Source: CAD feature listing. Evaluate the final solid. Frame: model axes, mm. Face numbers are marked on the shaded views. A direction names the side the tool comes from. Coordinates: 2 decimals unless noted, no trailing zeros. Write each loop counter-clockwise with the first axis right and the second up, starting at its lowest first coordinate (ties: lowest second). Pieces come first, ordered by that corner, then holes. Notation, with made-up numbers: M -36.75,11 L 0.25,11 A20 ccw 0.25,50 Z; hole C -36,50.5 d10. An arc over 180 degrees is marked long. Write item = value, one per line. Start each with the question number.
1. Pull-direction query (Y, two-part tool) for the marked faces 4, 5 and 6; classes: pulls with the +Y half, pulls with the -Y half, needs draft (parallel to the pull), parting line crosses it, or undercut.
2. Section query C-C (x = -10.5). Output: boundary loops of the cut face in (y, z), then the cut area to 3 significant figures.
3. Pin query (flat end, axial travel): pin 1 Ø5 at (x, z) = (-30, -24) entering from -Y; pin 2 Ø8 at (y, z) = (23.5, 6) entering from -X; pin 3 Ø3 at (x, z) = (-31, 23.5) entering from +Y; pin 4 Ø7 at (x, z) = (-9, -25.5) entering from +Y. Return the tip coordinate at first contact, or that it passes through.
4. Line query: line 1 along Z through (x, y) = (-10, -1); line 2 along Z through (x, y) = (5, 9.05); line 3 along Z through (x, y) = (-10, -5). Output: solid intervals per line, ascending.
5. Section query D-D (x = -5). Output: boundary loops of the cut face in (y, z), then the cut area to 3 significant figures.
6. Access query for the marked faces 1, 2 and 3. Directions: +Z, -Z, +X, -X, +Y, -Y. A direction counts if a zero-diameter tool reaches every point of the face in a straight line with its end or side. Return the directions, or none.
7. Section query B-B (y = 14). Output: boundary loops of the cut face in (x, z).
8. Section query A-A (z = -6). Output: boundary loops of the cut face in (x, y), then the cut area to 3 significant figures.
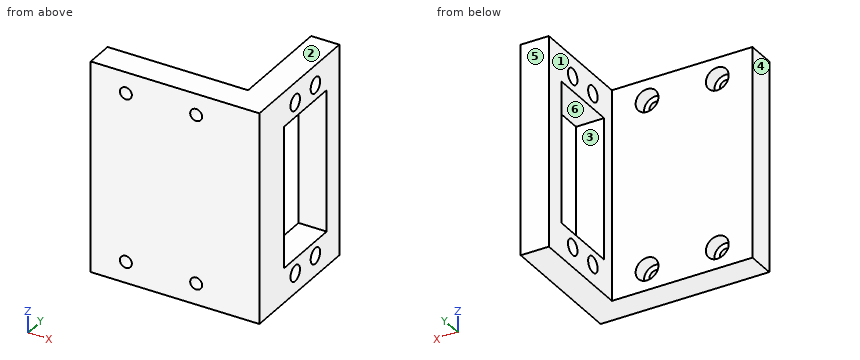
```python
from build123d import *

# Parameters (mm, degrees)
CROQUIS1_W                                 = 40
CROQUIS1_H                                 = 8
SALIENTE_EXTRUIR1_DEPTH                    = 30
CROQUIS2_W                                 = 40.3
CROQUIS2_H                                 = 20.3
CORTAR_EXTRUIR1_DEPTH                      = 60
CROQUIS3_R                                 = 2.25
CROQUIS3_W                                 = 40.3
CROQUIS3_H                                 = 20.3
CORTAR_EXTRUIR2_DEPTH                      = 60
CROQUIS4_R                                 = 3.25
CORTAR_EXTRUIR3_DEPTH                      = 4
TALADRO_DE_MARGEN_PARA_M31_D               = 3.4
TALADRO_DE_MARGEN_PARA_M31_DEPTH           = 11.5
TALADRO_DE_MARGEN_PARA_M31_TIP             = 1.021463052
TALADRO_DE_MARGEN_PARA_M31_ON_FACE_2_D     = 3.4
TALADRO_DE_MARGEN_PARA_M31_ON_FACE_2_DEPTH = 11.5
TALADRO_DE_MARGEN_PARA_M31_ON_FACE_2_TIP   = 1.021463052


with BuildPart() as part:
    # Croquis1 → Saliente-Extruir1 (new, symmetric)
    with BuildSketch(Plane.XY):
        with Locations((-20, -4)):
            Rectangle(CROQUIS1_W, CROQUIS1_H)
        Polygon((0, 30), (0, 0), (0, -8), (8, -8), (8, 30), align=None)
    extrude(amount=SALIENTE_EXTRUIR1_DEPTH, both=True)

    # Croquis2 → Cortar-Extruir1 (cut)
    with BuildSketch(Plane(origin=(8, 0, 0), x_dir=(0, 0, -1), z_dir=(1, 0, 0))):
        with Locations((0, 13.85)):
            Rectangle(CROQUIS2_W, CROQUIS2_H)
    extrude(amount=-CORTAR_EXTRUIR1_DEPTH, mode=Mode.SUBTRACT)

    # Croquis3 → Cortar-Extruir2 (cut)
    with BuildSketch(Plane(origin=(8, 0, 0), x_dir=(0, 0, -1), z_dir=(1, 0, 0))):
        with Locations(Location((-24.31, 18.65, 0), (0, 0, 90))):
            Circle(CROQUIS3_R)
        with Locations(Location((-24.31, 9.05, 0), (0, 0, 270))):
            Circle(CROQUIS3_R)
        with Locations(Location((24.31, 9.05, 0), (0, 0, 90))):
            Circle(CROQUIS3_R)
        with Locations(Location((24.31, 18.65, 0), (0, 0, 270))):
            Circle(CROQUIS3_R)
        with Locations((0, 13.85)):
            Rectangle(CROQUIS3_W, CROQUIS3_H)
    extrude(amount=-CORTAR_EXTRUIR2_DEPTH, mode=Mode.SUBTRACT)

    # Croquis4 → Cortar-Extruir3 (cut)
    with BuildSketch(Plane(origin=(0, 0, 0), x_dir=(1, 0, 0), z_dir=(0, 1, 0))):
        with Locations(Location((-30, 24, 0), (0, 0, 180))):
            Circle(CROQUIS4_R)
        with Locations((-10, 24)):
            Circle(CROQUIS4_R)
        with Locations(Location((-10, -24, 0), (0, 0, 180))):
            Circle(CROQUIS4_R)
        with Locations((-30, -24)):
            Circle(CROQUIS4_R)
    extrude(amount=-CORTAR_EXTRUIR3_DEPTH, mode=Mode.SUBTRACT)

    # Taladro de margen para M31
    with Locations(Plane(origin=(-30, -4, -24), x_dir=(1, 0, 0), z_dir=(0, 1, 0))):
        with Locations((0, 0), (20, 0), (0, -48)):
            Hole(TALADRO_DE_MARGEN_PARA_M31_D / 2, depth=TALADRO_DE_MARGEN_PARA_M31_DEPTH)
            with Locations((0, 0, -(TALADRO_DE_MARGEN_PARA_M31_DEPTH + TALADRO_DE_MARGEN_PARA_M31_TIP / 2))):  # 118° drill point
                Cone(0, TALADRO_DE_MARGEN_PARA_M31_D / 2, TALADRO_DE_MARGEN_PARA_M31_TIP, mode=Mode.SUBTRACT)

    # Taladro de margen para M31 on face 2
    with Locations(Plane(origin=(-10, 0, 24), x_dir=(1, 0, 0), z_dir=(0, 1, 0))):
        with Locations((0, 0)):
            Hole(TALADRO_DE_MARGEN_PARA_M31_ON_FACE_2_D / 2, depth=TALADRO_DE_MARGEN_PARA_M31_ON_FACE_2_DEPTH)
            with Locations((0, 0, -(TALADRO_DE_MARGEN_PARA_M31_ON_FACE_2_DEPTH + TALADRO_DE_MARGEN_PARA_M31_ON_FACE_2_TIP / 2))):  # 118° drill point
                Cone(0, TALADRO_DE_MARGEN_PARA_M31_ON_FACE_2_D / 2, TALADRO_DE_MARGEN_PARA_M31_ON_FACE_2_TIP, mode=Mode.SUBTRACT)


solid = part.part
```
Results are:
q1.face_4 = needs draft
q1.face_5 = pulls with the +Y half
q1.face_6 = undercut
q2.outline = M -8,-30 L 0,-30 L 0,-27.21 L -4,-27.21 L -4,-25.62 L -8,-25.62 Z; M -8,-22.38 L -4,-22.38 L -4,-20.79 L 0,-20.79 L 0,20.79 L -4,20.79 L -4,22.38 L -8,22.38 Z; M -8,25.62 L -4,25.62 L -4,27.21 L 0,27.21 L 0,30 L -8,30 Z
q2.area = 403 mm^2
q3.pin_1 = -8
q3.pin_2 = 0
q3.pin_3 = -4
q3.pin_4 = 0
q4.line_1 = -30 to -27.25, -20.75 to 20.75, 27.25 to 30
q4.line_2 = -30 to -26.56, -22.06 to -20.15, 20.15 to 22.06, 26.56 to 30
q4.line_3 = -30 to -25.7, -22.3 to 22.3, 25.7 to 30
q5.outline = M -8,-30 L 0,-30 L 0,30 L -8,30 Z
q5.area = 480 mm^2
q6.face_1 = +Z, -Z, -X, +Y
q6.face_2 = +Z, +X, -X, +Y, -Y
q6.face_3 = +X, -X
q7.outline = M 0,-30 L 8,-30 L 8,-20.15 L 0,-20.15 Z; M 0,20.15 L 8,20.15 L 8,30 L 0,30 Z
q8.outline = M -40,-8 L 8,-8 L 8,3.7 L 0,3.7 L 0,0 L -40,0 Z; M 0,24 L 8,24 L 8,30 L 0,30 Z
q8.area = 462 mm^2
